```python
from build123d import *

# Parameters (mm, degrees)
SKETCH1_W           = 71.7
SKETCH1_H           = 56.7
BOSS_EXTRUDE1_DEPTH = 5
SKETCH2_W           = 68.5
SKETCH2_H           = 53.5
SKETCH2_W_2         = 66.5
SKETCH2_H_2         = 51.5
BOSS_EXTRUDE2_DEPTH = 2
SKETCH2_2_W         = 66.5
SKETCH2_2_H         = 51.5
CUT_EXTRUDE1_DEPTH  = 4
SKETCH3_R           = 2.5
SKETCH3_R_2         = 10
CUT_EXTRUDE2_DEPTH  = 1


with BuildPart() as part:
    # Sketch1 → Boss-Extrude1 (new body)
    with BuildSketch(Plane(origin=(0, 0, 0), x_dir=(1, 0, 0), z_dir=(0, 1, 0))):
        with Locations((11.345000373, -6.211960564)):
            Rectangle(SKETCH1_W, SKETCH1_H)
    extrude(amount=BOSS_EXTRUDE1_DEPTH)

    # Sketch2 → Boss-Extrude2 (add)
    with BuildSketch(Plane.XZ):
        with Locations((11.345000373, 6.211960564)):
            Rectangle(SKETCH2_W, SKETCH2_H)
        with Locations((11.345000373, 6.211960564)):
            Rectangle(SKETCH2_W_2, SKETCH2_H_2, mode=Mode.SUBTRACT)
    extrude(amount=BOSS_EXTRUDE2_DEPTH)

    # Sketch2_2 → Cut-Extrude1 (cut)
    with BuildSketch(Plane.XZ):
        with Locations((11.345000373, 6.211960564)):
            Rectangle(SKETCH2_2_W, SKETCH2_2_H)
    extrude(amount=-CUT_EXTRUDE1_DEPTH, mode=Mode.SUBTRACT)

    # Sketch3 → Cut-Extrude2 (cut)
    with BuildSketch(Plane(origin=(0, 5, 0), x_dir=(1, 0, 0), z_dir=(0, 1, 0))):
        with Locations(Location((-17.004999627, -24.561960564, 0), (0, 0, 270))):
            Circle(SKETCH3_R)
        with Locations(Location((-17.004999627, -17.061960564, 0), (0, 0, 270))):
            Circle(SKETCH3_R)
        with Locations(Location((-17.004999627, -9.561960564, 0), (0, 0, 270))):
            Circle(SKETCH3_R)
        with Locations(Location((11.345000373, -6.211960564, 0), (0, 0, 270))):
            Circle(SKETCH3_R_2)
    extrude(amount=-CUT_EXTRUDE2_DEPTH, mode=Mode.SUBTRACT)


solid = part.part
```
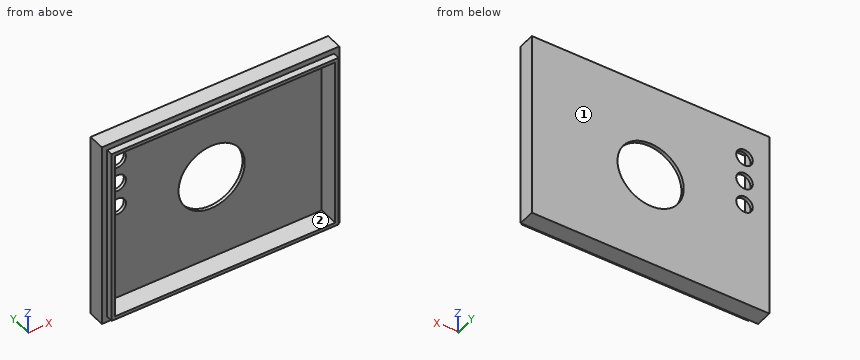
Model file for the job. Use its own axes, mm. Face numbers are marked on the shaded views. Round coordinates to 2 decimals unless told otherwise and drop trailing zeros. Write each loop counter-clockwise with the first axis right and the second up, starting at its lowest first coordinate (ties: lowest second). Pieces come first, ordered by that corner, then holes. Notation, with made-up numbers: M 58,48.25 L 98,48.25 A23 cw 98,87.25 Z; hole C 51,24 d1. An arc over 180 degrees is marked long. Put each result on its own line as item: value.
Item 1: Cut at C-C (z = -2). List the corners of the cut face in (x, y) (3 decimals).
Responses:
outline: M -24.505,0 L -22.905,0 L -22.905,-2 L -21.905,-2 L -21.905,4 L 5.639,4 L 5.639,5 L -24.505,5 Z; M 17.051,4 L 44.595,4 L 44.595,-2 L 45.595,-2 L 45.595,0 L 47.195,0 L 47.195,5 L 17.051,5 Z
Item 2: Mould opens along Z. For the marked faces 1 and 2 say: +Z half, -Z half, draft (parallel to the pull), parting line (faces both ways), or undercut.
Responses:
face 1: draft
face 2: undercut
Item 3: Cut at D-D (x = 17). List the corners of the cut face in (y, z).
Responses:
outline: M -2,-20.54 L 0,-20.54 L 0,-22.14 L 5,-22.14 L 5,-2.04 L 4,-2.04 L 4,-19.54 L -2,-19.54 Z; M -2,31.96 L 4,31.96 L 4,14.46 L 5,14.46 L 5,34.56 L 0,34.56 L 0,32.96 L -2,32.96 Z
Item 4: Probe L1, parallel to Z at x = 8.5, y = -1.25; L2, parallel to X at y = -1.5, z = -5.5 (3 decimals); L3, parallel to Z at x = 11, y = 1.25. List the from-to ranges inside material, lowest first. Write a range as from..to.
Responses:
L1: -20.54..-19.54, 31.96..32.96
L2: -22.905..-21.905, 44.595..45.595
L3: -22.14..-19.54, 31.96..34.56
Item 5: Cut at B-B (x = -10.5). List the corners of the cut face in (y, z), and give its area (3 significant figures).
Responses:
outline: M -2,-20.54 L 0,-20.54 L 0,-22.14 L 5,-22.14 L 5,34.56 L 0,34.56 L 0,32.96 L -2,32.96 L -2,31.96 L 4,31.96 L 4,-19.54 L -2,-19.54 Z
area: 81.5 mm²
Item 6: Cut at A-A (y = 3.25). List the corners of the cut face in (x, z) (3 decimals), and give its area (3 significant figures).
Responses:
outline: M -24.505,-22.138 L 47.195,-22.138 L 47.195,34.562 L -24.505,34.562 Z; hole M -21.905,-19.538 L 44.595,-19.538 L 44.595,31.962 L -21.905,31.962 Z
area: 641 mm²
Item 7: Flat gauge pins, fed straight in: P1, Ø4, axis at x = 12.5, z = -9.5, coming from the -Y side; P2, Ø1, axis at y = -1, z = -6, coming from the +X side (3 decimals); P3, Ø1.6, axis at y = -1, z = 13.5, coming from the -X side (3 decimals). Where does each tip first touch, or does it go through?
Responses:
P1: y = 4
P2: x = 45.595
P3: x = -22.905
